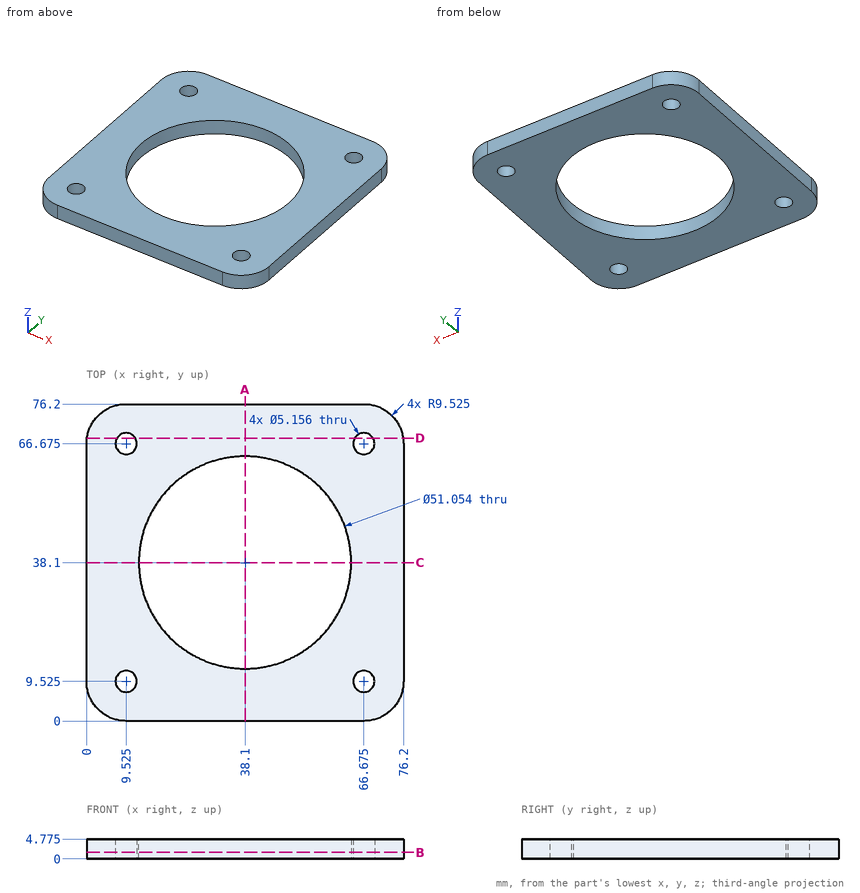
Part print with two shaded views. Sizes in mm from the minimum x, y, z corner. Round coordinates to 2 decimals unless told otherwise and drop trailing zeros. Order: outer loops, then holes, each group sorted by start corner. A loop starts at its lowest first (then second) coordinate and runs counter-clockwise, first axis right, second up. Notation, with made-up numbers: (39, 21.5) -> (55, 21.5) arc R14 cw to (55, 40.5) -> close; hole circle Ø9 at (35, 79.25). An arc over 180 degrees is marked (long way). Write each question's results on one line, items separated by ' | '.
1. Cut at B-B (z = 1.55). Count the separate pieces of the cut face and the enclosed holes in it, plus the area to 3 significant figures.
Findings below:
separate pieces: 1 | enclosed holes: 5 | area: 3,600 mm²
2. Wall check: line 1 along X through (y, z) = (9.5, 2.8); line 2 along Y through (x, z) = (38, 2.3). Give the ranges that are in metal, low to high. Write a range as [from, to].
Findings below:
line 1: x = [0, 6.95], [12.1, 64.1], [69.25, 76.2] | line 2: y = [0, 12.57], [63.63, 76.2]
3. Cut at D-D (y = 68). Give the cut face in (x, z) (1 decimal).
Findings below:
outline: (0.1, 0) -> (7.3, 0) -> (7.3, 4.8) -> (0.1, 4.8) -> close; (11.7, 0) -> (64.5, 0) -> (64.5, 4.8) -> (11.7, 4.8) -> close; (68.9, 0) -> (76.1, 0) -> (76.1, 4.8) -> (68.9, 4.8) -> close
4. Cut at A-A (x = 38.1). Give the cut face in (y, z) (1 decimal), plus the area to 3 significant figures.
Findings below:
outline: (0, 0) -> (12.6, 0) -> (12.6, 4.8) -> (0, 4.8) -> close; (63.6, 0) -> (76.2, 0) -> (76.2, 4.8) -> (63.6, 4.8) -> close | area: 120 mm²
